```python
from build123d import *

# Parameters (mm, degrees)
ESBO_O1_R                = 12.5
ESBO_O1_R_2              = 2
RESSALTO_EXTRUS_O1_DEPTH = 6
RESSALTO_EXTRUS_O2_DEPTH = 20
ESBO_O3_R                = 4.15
RESSALTO_EXTRUS_O3_DEPTH = 8
ESBO_O5_R                = 1.75
ESBO_O5_R_2              = 4.15
CORTE_EXTRUS_O2_DEPTH    = 12
ESBO_O6_R                = 1.75
CORTE_EXTRUS_O3_DEPTH    = 12
CHANFRO1_SIZE            = 5
ESBO_O8_R                = 5.25
CORTE_EXTRUS_O5_DEPTH    = 1
ESBO_O9_R                = 5.25
CORTE_EXTRUS_O6_DEPTH    = 1


with BuildPart() as part:
    # Esboço1 → Ressalto-extrusão1 (new body)
    with BuildSketch(Plane.XY):
        Polygon((-44, 7), (-21, -21), (21, -21), (21, 21), (11, 29), (-24, 29), (-24, 21), (-24, 11), (-44, 11), align=None)
        Circle(ESBO_O1_R, mode=Mode.SUBTRACT)
        with Locations((15.5, 15.5)):
            Circle(ESBO_O1_R_2, mode=Mode.SUBTRACT)
        with Locations((15.5, -15.5)):
            Circle(ESBO_O1_R_2, mode=Mode.SUBTRACT)
        with Locations((-15.5, -15.5)):
            Circle(ESBO_O1_R_2, mode=Mode.SUBTRACT)
    extrude(amount=RESSALTO_EXTRUS_O1_DEPTH)

    # Esboço2 → Ressalto-extrusão2 (add)
    with BuildSketch(Plane(origin=(0, 0, 0), x_dir=(-1, 0, 0), z_dir=(0, 0, -1))):
        with BuildLine():
            Line((44, 11), (44, 7))
            Line((44, 7), (24, 7))
            ThreePointArc((24, 7), (21.171572875, 8.171572875), (20, 11))
            Line((20, 11), (20, 29))
            Line((20, 29), (24, 29))
            Line((24, 29), (24, 11))
            Line((24, 11), (44, 11))
        make_face()
    extrude(amount=RESSALTO_EXTRUS_O2_DEPTH)

    # Esboço3 → Ressalto-extrusão3 (add)
    with BuildSketch(Plane(origin=(-20, 0, 0), x_dir=(0, 0, -1), z_dir=(1, 0, 0))):
        Polygon((0, 29), (8, 29), (12.5, 24.5), (12.5, 13.5), (8, 9), (0, 9), align=None)
        with Locations((6, 19)):
            Circle(ESBO_O3_R, mode=Mode.SUBTRACT)
    extrude(amount=RESSALTO_EXTRUS_O3_DEPTH)

    # Esboço5 → Corte-extrusão2 (cut)
    with BuildSketch(Plane(origin=(-20, 0, 0), x_dir=(0, 0, -1), z_dir=(1, 0, 0))):
        with Locations((16, 21)):
            Circle(ESBO_O5_R)
        with Locations((6, 19)):
            Circle(ESBO_O5_R_2)
    extrude(amount=-CORTE_EXTRUS_O2_DEPTH, mode=Mode.SUBTRACT)

    # Esboço6 → Corte-extrusão3 (cut)
    with BuildSketch(Plane(origin=(0, 7, 0), x_dir=(-1, 0, 0), z_dir=(0, -1, 0))):
        with Locations((34.5, 13)):
            Circle(ESBO_O6_R)
    extrude(amount=-CORTE_EXTRUS_O3_DEPTH, mode=Mode.SUBTRACT)

    # Chanfro1
    chanfro1_edges = [part.edges().sort_by_distance(p)[0] for p in [
        (21, -21, 3),
    ]]
    chamfer(chanfro1_edges, length=CHANFRO1_SIZE)

    # Esboço8 → Corte-extrusão5 (cut)
    with BuildSketch(Plane.ZY.offset(24)):
        with Locations((-16, 21)):
            Circle(ESBO_O8_R)
    extrude(amount=-CORTE_EXTRUS_O5_DEPTH, mode=Mode.SUBTRACT)

    # Esboço9 → Corte-extrusão6 (cut)
    with BuildSketch(Plane(origin=(0, 11, 0), x_dir=(1, 0, 0), z_dir=(0, 1, 0))):
        with Locations((-34.5, 13)):
            Circle(ESBO_O9_R)
    extrude(amount=-CORTE_EXTRUS_O6_DEPTH, mode=Mode.SUBTRACT)


solid = part.part
```
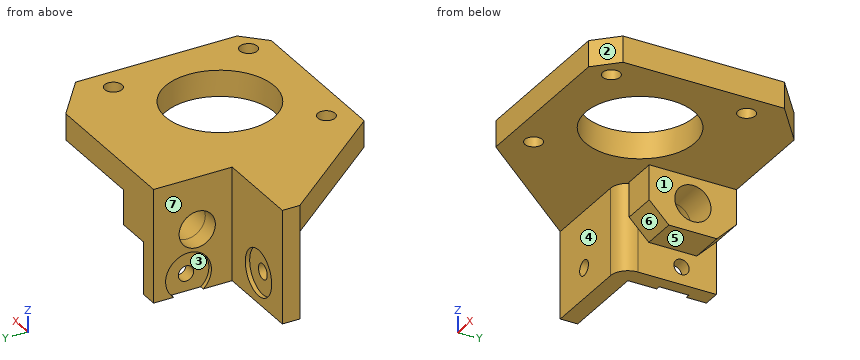
The model under review builds one solid part; all positions refer to its coordinate system, in mm. Face numbers are marked on the shaded views. A direction names the side the tool comes from. Round coordinates to 2 decimals unless told otherwise and drop trailing zeros. Loops run counter-clockwise (first coordinate to the right, second up) from the corner with the lowest first, then second, coordinate; pieces in that order, holes last. Notation, with made-up numbers: (46.25, -2.75) -> (55.25, -2.75) arc R30 ccw to (55.25, 31.25) -> close; hole circle Ø11 at (-34, -9). An arc over 180 degrees is marked (long way). Answer in a Markdown table with one row per item.
1) Draft analysis for pull direction Y (two halves, no side actions). For the marked faces 1, 2 and 3, state which applies: pulls with the +Y half, pulls with the -Y half, needs draft (parallel to the pull), parting line crosses it, or undercut.
Taken from the geometry:
| item | result |
|---|---|
| face 1 | needs draft |
| face 2 | pulls with the -Y half |
| face 3 | undercut |
2) Tool access review of the marked faces 4, 5, 6 and 7: name each direction out of +Z, -Z, +X, -X, +Y, -Y from which nothing blocks a thin tool from reaching the whole face with its end or side.
Taken from the geometry:
| item | result |
|---|---|
| face 4 | -Z, +X, -X, -Y |
| face 5 | -Z, +X, +Y, -Y |
| face 6 | -Z, +X, -Y |
| face 7 | +Z, -Z, -X, +Y |
3) Wall thickness on line 1 along Y through (x, z) = (-15.5, 3.75); line 2 along Y through (x, z) = (15.5, 1.9); line 3 along Z through (x, y) = (-34.5, 7.8): over which ranges is each line inside the solid? List them lowest first.
Taken from the geometry:
| item | result |
|---|---|
| line 1 | y = -21 to -17.5, -13.5 to 29 |
| line 2 | y = -21 to -17.5, -13.5 to 13.5, 17.5 to 25.4 |
| line 3 | z = -20 to -14.75, -11.25 to 6 |
4) For pin 1 Ø4 at (y, z) = (15, -3.5) entering from +X; pin 2 Ø1 at (x, z) = (-32, 1) entering from +Y; pin 3 Ø8 at (y, z) = (1.5, -14.5) entering from -X; pin 4 Ø5 at (y, z) = (18, -2) entering from -X, all flat-tipped, find the tip position at first contact; note any pin that passes through.
Taken from the geometry:
| item | result |
|---|---|
| pin 1 | stops at x = -12 |
| pin 2 | stops at y = 11 |
| pin 3 | passes through |
| pin 4 | stops at x = -24 |
5) Consider section C-C, the plane z = -6. Write out the cut boundary in (x, y), plus the area to 3 significant figures.
Taken from the geometry:
| item | result |
|---|---|
| outline | (-44, 7) -> (-24, 7) arc R4 ccw to (-20, 11) -> (-20, 9) -> (-12, 9) -> (-12, 14.85) -> (-24, 14.85) -> (-24, 11) -> (-44, 11) -> close; (-24, 23.15) -> (-12, 23.15) -> (-12, 29) -> (-24, 29) -> close |
| area | 225 mm² |
6) Consider section A-A, the plane x = -15.5. Write out the cut boundary in (y, z), plus the area to 3 significant figures.
Taken from the geometry:
| item | result |
|---|---|
| outline | (-21, 0) -> (-17.5, 0) -> (-17.5, 6) -> (-21, 6) -> close; (-13.5, 0) -> (9, 0) -> (9, -8) -> (13.5, -12.5) -> (24.5, -12.5) -> (29, -8) -> (29, 6) -> (-13.5, 6) -> close; hole circle Ø8.3 at (19, -6) |
| area | 452 mm² |
7) Consider section D-D, the plane x = 0. Write out the cut boundary in (y, z), plus the area to 3 significant figures.
Taken from the geometry:
| item | result |
|---|---|
| outline | (-21, 0) -> (-12.5, 0) -> (-12.5, 6) -> (-21, 6) -> close; (12.5, 0) -> (29, 0) -> (29, 6) -> (12.5, 6) -> close |
| area | 150 mm² |
8) Consider section B-B, the plane y = 0. Write out the cut boundary in (x, z).
Taken from the geometry:
| item | result |
|---|---|
| outline | (-38.25, 0) -> (-12.5, 0) -> (-12.5, 6) -> (-38.25, 6) -> close; (12.5, 0) -> (21, 0) -> (21, 6) -> (12.5, 6) -> close |
